For this review, take the finished solid that the model builds, in its own axes (mm). A direction names the side the tool comes from. Coordinates: 2 decimals unless noted, no trailing zeros. Order: outer loops, then holes, each group sorted by start corner. A loop starts at its lowest first (then second) coordinate and runs counter-clockwise, first axis right, second up. Notation, with made-up numbers: (63.25, 78) -> (77.25, 78) arc R9 ccw to (77.25, 88) -> close; hole circle Ø10 at (56, 22). An arc over 180 degrees is marked (long way). Answer as a JSON object with one key per item and string values. Group by question number.
1) Machinability: for faces 1 (the flat face through (75, 26, 0)), 2 (the cylindrical face through (74.235, 34.072, 6.266)), 3 (the flat face through (126, -21, 18)), 4 (the cylindrical face through (21, -15, -12)), 5 (the conical face through (54.879, -25.711, 27.465)), which of the approach directions +Z, -Z, +X, -X, +Y, -Y give a long, thin tool a straight path to every point of the face, cutting with its end or side? Answer none if there is none.
2) Wall thickness on L1, parallel to Y at x = 76, z = 32; L2, parallel to Z at x = 31, y = -25.5; L3, parallel to Y at x = 72, z = 26: over which ranges is each line inside the solid? List them lowest first.
3) Draft analysis for pull direction Y (two halves, no side actions). For faces 6 (the cylindrical face through (74.235, -34.374, 9.718)), 7 (the conical face through (92.156, -25.734, 27.491)), 8 (the cylindrical face through (74.235, -19.465, 20.611)), 9 (the flat face through (147, -6, 5)), state which applies: +Y half, -Y half, draft (parallel to the pull), parting line (faces both ways), or undercut.
4) Add section B-B, the plane x = 62. Count the separate pieces of the cut face and the enclosed holes in it, then the cut area to 3 significant figures.
5) For pin 1 (13 mm diameter, centred on x = 82.5, z = 7, fed in from -Y); pin 2 (8.5 mm diameter, centred on y = 22.63, z = 22.63, fed in from +X); pin 3 (7 mm diameter, centred on y = -30.91, z = 8.28, fed in from -X); pin 4 (1 mm diameter, centred on x = 36.5, y = -22, fed in from -Z), all flat-tipped, find the tip position at first contact; note any pin that passes through.
6) Add section A-A, the plane x = 135. Write out the cut boundary in (y, z), then the cut area to 3 significant figures.
from build123d import *

# Parameters (mm, degrees)
CONG_1_R                     = 2
ENL_V_MAT_EXTRU_1_DEPTH      = 158.508729917
ENL_V_MAT_EXTRU_2_DEPTH      = 158.508729917
ESQUISSE6_R                  = 3.75
ENL_V_MAT_EXTRU_4_DEPTH      = 139.115893365
R_P_TITION_CIRCULAIRE1_COUNT = 9
R_P_TITION_CIRCULAIRE1_ANGLE = 240
ENL_V_MAT_EXTRU_5_DEPTH      = 80


with BuildPart() as part:
    # Esquisse1 → Révolution1 (revolve)
    with BuildSketch(Plane.XY, mode=Mode.PRIVATE) as r_volution1_sk:
        Polygon((0, 0), (0, 25), (21, 25), (21, 40), (52.5, 40), (55, 37.5), (92, 37.5), (94.5, 40), (126, 40), (126, 25), (147, 25), (147, 0), align=None)
    revolve(r_volution1_sk.sketch.rotate(Axis((0, 0, 0), (1, 0, 0)), 90), axis=Axis((0, 0, 0), (1, 0, 0)))

    # Congé1
    cong_1_edges = [part.edges().sort_by_distance(p)[0] for p in [
        (126, 0, -25),
        (21, 0, -25),
    ]]
    fillet(cong_1_edges, radius=CONG_1_R)

    # Esquisse3 → Enlèv. mat.-Extru.1 (cut, through all)
    with BuildSketch(Plane(origin=(147, 0, 0), x_dir=(0, 0, -1), z_dir=(1, 0, 0))):
        with BuildLine():
            Line((0, 0), (0, 40))
            ThreePointArc((0, 40), (28.284271247, 28.284271247), (40, 0))
            Line((40, 0), (0, 0))
        make_face()
    extrude(amount=-ENL_V_MAT_EXTRU_1_DEPTH, mode=Mode.SUBTRACT)

    # Esquisse4 → Enlèv. mat.-Extru.2 (cut, through all)
    with BuildSketch(Plane(origin=(147, 0, 0), x_dir=(0, 0, -1), z_dir=(1, 0, 0))):
        with BuildLine():
            Line((12, 7), (-12, 7))
            ThreePointArc((-12, 7), (-15, 10), (-12, 13))
            Line((-12, 13), (12, 13))
            ThreePointArc((12, 13), (15, 10), (12, 7))
        make_face()
    extrude(amount=-ENL_V_MAT_EXTRU_2_DEPTH, mode=Mode.SUBTRACT)

    # Esquisse6 → Enlèv. mat.-Extru.4 (cut, through all)
    with BuildSketch(Plane(origin=(126, 0, 0), x_dir=(0, 0, -1), z_dir=(1, 0, 0))):
        with Locations((-8.282209443, 30.909626441)):
            Circle(ESQUISSE6_R)
    enl_v_mat_extru_4 = extrude(amount=-ENL_V_MAT_EXTRU_4_DEPTH, mode=Mode.SUBTRACT)

    # Répétition circulaire1: Enlèv. mat.-Extru.4 ×9 about axis
    r_p_tition_circulaire1_axis = Axis((0, 0, 0), (1, 0, 0))
    for i in range(1, R_P_TITION_CIRCULAIRE1_COUNT):
        add(enl_v_mat_extru_4.rotate(r_p_tition_circulaire1_axis, i * R_P_TITION_CIRCULAIRE1_ANGLE / (R_P_TITION_CIRCULAIRE1_COUNT - 1)), mode=Mode.SUBTRACT)

    # Esquisse7 → Enlèv. mat.-Extru.5 (cut)
    with BuildSketch(Plane(origin=(0, 0, 0), x_dir=(1, 0, 0), z_dir=(0, 1, 0))):
        with BuildLine():
            Line((30, 40), (0, 40))
            Line((0, 40), (0, 10))
            ThreePointArc((0, 10), (2.614672282, 10.114159057), (5.20944533, 10.45576741))
            Line((5.20944533, 10.45576741), (6.077686218, 5.531728645))
            ThreePointArc((6.077686218, 5.531728645), (21.306650015, 12.23263309), (31.720772546, 25.208360839))
            Line((31.720772546, 25.208360839), (27.189233611, 27.321452148))
            ThreePointArc((27.189233611, 27.321452148), (29.288880214, 33.506811582), (30, 40))
        make_face()
    extrude(amount=-ENL_V_MAT_EXTRU_5_DEPTH, mode=Mode.SUBTRACT)


solid = part.part
Output values:
{
 "1": {"face 1": "-Z, +X, -X, +Y", "face 2": "+X, -X", "face 3": "+X", "face 4": "+Y, -Y", "face 5": "none"},
 "2": {"L1": "y = -19.55 to -11.87, -4.69 to 4.69, 11.87 to 19.55", "L2": "z = -30.82 to -25.54, -20.22 to 20.22, 25.04 to 30.82", "L3": "y = -27.02 to -24.27, -20.99 to 20.99, 24.27 to 27.02"},
 "3": {"face 6": "undercut", "face 7": "parting line", "face 8": "undercut", "face 9": "draft"},
 "4": {"separate pieces": "1", "enclosed holes": "9", "area": "2,830 mm²"},
 "5": {"pin 1": "stops at y = -37.5", "pin 2": "stops at x = 126", "pin 3": "passes through", "pin 4": "stops at z = -33.73"},
 "6": {"outline": "(0, -25) -> (0, 0) -> (7, 0) -> (7, 12) arc R3 cw to (13, 12) -> (13, 0) -> (25, 0) arc R25 ccw (long way) to start", "area": "1,390 mm²"}
}
